```python
from build123d import *

# Parameters (mm, degrees)
CROQUIS1_R                 = 1.5
CROQUIS1_W                 = 20
CROQUIS1_H                 = 10.5
SALIENTE_EXTRUIR1_DEPTH    = 10
CORTAR_EXTRUIR1_REACH      = 72.33
CROQUIS2_W                 = 10
CROQUIS2_H                 = 10
CROQUIS5_W                 = 15
CROQUIS5_H                 = 10.5
CORTAR_EXTRUIR5_DEPTH      = 10
CORTAR_EXTRUIR4_DEPTH      = 62.923844357
CORTAR_EXTRUIR4_DEPTH_BACK = 62.923844357
CROQUIS4_W                 = 15
CROQUIS4_H                 = 2
CORTAR_EXTRUIR3_REACH      = 47.503
CROQUIS3_W                 = 8.3
CROQUIS3_H                 = 23
REDONDEO2_R                = 1


with BuildPart() as part:
    # Croquis1 → Saliente-Extruir1 (new, symmetric)
    with BuildSketch(Plane(origin=(0, 0, 0), x_dir=(0, 0, -1), z_dir=(1, 0, 0))):
        Polygon((-58, 6.75), (-58, -19.25), (-18, -19.25), (-18, -11.75), (-18, 11.25), (-1.5, 11.25), (-1.5, 19.25), (-28, 19.25), (-28, 6.75), align=None)
        with Locations((-5, 15.25)):
            Circle(CROQUIS1_R, mode=Mode.SUBTRACT)
        with Locations((-38, -6.5)):
            Rectangle(CROQUIS1_W, CROQUIS1_H, mode=Mode.SUBTRACT)
    extrude(amount=SALIENTE_EXTRUIR1_DEPTH, both=True)

    # Cortar-Extruir1: up to this face of the body (flat: up to its plane)
    cortar_extruir1_end = Plane(part.part.faces().sort_by_distance((0, 11.25, 9.75))[0])
    # Croquis2 → Cortar-Extruir1 (cut, up to the picked face)
    with BuildSketch(Plane(origin=(0, 19.25, 0), x_dir=(1, 0, 0), z_dir=(0, 1, 0)), mode=Mode.PRIVATE) as cortar_extruir1_sk1:
        with Locations((0, -6.5)):
            Rectangle(CROQUIS2_W, CROQUIS2_H)
    cortar_extruir1_tool1 = split(extrude(cortar_extruir1_sk1.sketch, amount=-CORTAR_EXTRUIR1_REACH, mode=Mode.PRIVATE), bisect_by=cortar_extruir1_end, keep=Keep.BOTH, mode=Mode.PRIVATE)
    add(cortar_extruir1_tool1.solids().sort_by(Axis((0, 19.25, 6.5), (0, -1, 0)))[0], mode=Mode.SUBTRACT)

    # Croquis5 → Cortar-Extruir5 (cut)
    with BuildSketch(Plane.XY.offset(58)):
        with Locations((0, -6.5)):
            Rectangle(CROQUIS5_W, CROQUIS5_H)
    extrude(amount=-CORTAR_EXTRUIR5_DEPTH, mode=Mode.SUBTRACT)

    # Croquis4 → Cortar-Extruir4 (cut, two sides: drawn at the far end of the back side and taken through both)
    with BuildSketch(Plane(origin=(0, 0, 0), x_dir=(0, 0, -1), z_dir=(1, 0, 0)).offset(-CORTAR_EXTRUIR4_DEPTH_BACK)):
        with Locations((-48, -16.25)):
            Rectangle(CROQUIS4_W, CROQUIS4_H)
        with Locations((-28, -16.25)):
            Rectangle(CROQUIS4_W, CROQUIS4_H)
    extrude(amount=CORTAR_EXTRUIR4_DEPTH + CORTAR_EXTRUIR4_DEPTH_BACK, mode=Mode.SUBTRACT)

    # Cortar-Extruir3: up to this face of the body (flat: up to its plane)
    cortar_extruir3_end = Plane(part.part.faces().sort_by_distance((-8.75, -6.5, 48))[0])
    # Croquis3 → Cortar-Extruir3 (cut, up to the picked face)
    with BuildSketch(Plane.XY.offset(18), mode=Mode.PRIVATE) as cortar_extruir3_sk1:
        with Locations((0, -0.25)):
            Rectangle(CROQUIS3_W, CROQUIS3_H)
    cortar_extruir3_tool1 = split(extrude(cortar_extruir3_sk1.sketch, amount=CORTAR_EXTRUIR3_REACH, mode=Mode.PRIVATE), bisect_by=cortar_extruir3_end, keep=Keep.BOTH, mode=Mode.PRIVATE)
    add(cortar_extruir3_tool1.solids().sort_by(Axis((0, -0.25, 18), (0, 0, 1)))[0], mode=Mode.SUBTRACT)

    # Redondeo2
    redondeo2_edges = [part.edges().sort_by_distance(p)[0] for p in [
        (-10, -19.25, 38),
        (0, -19.25, 58),
        (0, -19.25, 18),
        (10, -19.25, 38),
    ]]
    fillet(redondeo2_edges, radius=REDONDEO2_R)


solid = part.part
```
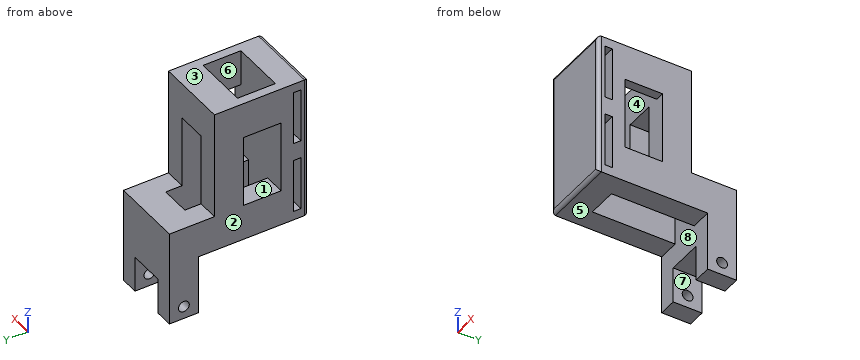
Work out the finished part from the listing and answer in its coordinate system (mm). Face numbers are marked on the shaded views. A direction names the side the tool comes from. Give positions to 0.01 mm unless a question says otherwise; leave off trailing zeros. Loops run counter-clockwise (first coordinate to the right, second up) from the corner with the lowest first, then second, coordinate; pieces in that order, holes last. Notation, with made-up numbers: (31, -37.5) -> (84, -37.5) arc R14 ccw to (84, -32.5) -> close; hole circle Ø6 at (26, -17.5). An arc over 180 degrees is marked (long way). Use CSV: the item, a comma, the result in double quotes.
1. The part is cut by section C-C (y = 15.25). Write down the section's boundary in (x, z), then the cut area to 3 significant figures.
Found:
outline,"(-10, 1.5) -> (-5, 1.5) -> (-5, 3.5) -> (-10, 3.5) -> close; (-10, 6.5) -> (-5, 6.5) -> (-5, 11.5) -> (5, 11.5) -> (5, 6.5) -> (10, 6.5) -> (10, 28) -> (-10, 28) -> close; (5, 1.5) -> (10, 1.5) -> (10, 3.5) -> (5, 3.5) -> close"
area,"400 mm^2"
2. A tool of negligible diameter and unlimited length cuts with its end or side. For the marked faces 4, 5, 6, 7 and 8, from which of +Z, -Z, +X, -X, +Y, -Y can it reach the whole face along a straight path? Write none if from no direction.
Found:
face 4,"none"
face 5,"-Z, +X, -X, -Y"
face 6,"+Z"
face 7,"-Z, +Y, -Y"
face 8,"-Z"
3. Flat-ended cylindrical pins translate along their axes: pin 1 Ø4 at (x, z) = (3.5, 48.5) entering from +Y; pin 2 Ø10 at (x, y) = (2, 1) entering from -Z; pin 3 Ø4 at (y, z) = (10, 47) entering from -X; pin 4 Ø5 at (x, y) = (0.5, 15.5) entering from -Z. Find the tip coordinate at first contact, or state that the pin passes through.
Found:
pin 1,"y = 6.75"
pin 2,"z = 18"
pin 3,"through"
pin 4,"z = 11.5"
4. The part is cut by section A-A (x = 2.25). Write down the section's boundary in (y, z), then the cut area to 3 significant figures.
Found:
outline,"(-19.25, 19) arc R1 ccw to (-18.25, 18) -> (-11.75, 18) -> (-11.75, 58) -> (-18.25, 58) arc R1 ccw to (-19.25, 57) -> close; (-1.25, 48) -> (6.75, 48) -> (6.75, 58) -> (-1.25, 58) -> close; (11.25, 11.5) -> (19.25, 11.5) -> (19.25, 28) -> (11.25, 28) -> close; hole (-17.25, 20.5) -> (-15.25, 20.5) -> (-15.25, 35.5) -> (-17.25, 35.5) -> close; hole (-17.25, 40.5) -> (-15.25, 40.5) -> (-15.25, 55.5) -> (-17.25, 55.5) -> close"
area,"452 mm^2"
5. Straight lines are drawn through the part: line 1 (Z direction, x = -7.5, y = 15.25); line 2 (Y direction, x = 1.75, z = 55); line 3 (Y direction, x = -7.2, z = 5). For each, find the intervals that lie inside material, in ascending order.
Found:
line 1,"1.5 to 3.5, 6.5 to 28"
line 2,"-19.25 to -17.25, -15.25 to -11.75, -1.25 to 6.75"
line 3,"11.25 to 13.75, 16.75 to 19.25"
6. The mould has two halves that part along Z. Classify the marked faces 1, 2 and 3: +Z half, -Z half, draft (parallel to the pull), parting line (faces both ways), or undercut.
Found:
face 1,"undercut"
face 2,"draft"
face 3,"+Z half"
7. The part is cut by section D-D (z = 53.5). Write down the section's boundary in (x, y), then the cut area to 3 significant figures.
Found:
outline,"(-10, -18.25) arc R1 ccw to (-9, -19.25) -> (9, -19.25) arc R1 ccw to (10, -18.25) -> (10, -17.25) -> (-10, -17.25) -> close; (-10, -15.25) -> (10, -15.25) -> (10, 6.75) -> (-10, 6.75) -> close; hole (-7.5, -11.75) -> (7.5, -11.75) -> (7.5, -1.25) -> (-7.5, -1.25) -> close"
area,"322 mm^2"
8. The part is cut by section B-B (z = 29.5). Write down the section's boundary in (x, y), then the cut area to 3 significant figures.
Found:
outline,"(-10, -18.25) arc R1 ccw to (-9, -19.25) -> (9, -19.25) arc R1 ccw to (10, -18.25) -> (10, -17.25) -> (-10, -17.25) -> close; (-10, -15.25) -> (10, -15.25) -> (10, -11.75) -> (-10, -11.75) -> close; (-10, -1.25) -> (-4.15, -1.25) -> (-4.15, 6.75) -> (-10, 6.75) -> close; (4.15, -1.25) -> (10, -1.25) -> (10, 6.75) -> (4.15, 6.75) -> close"
area,"203 mm^2"
